The listing builds one solid part. Answer for the finished solid, in the listing's coordinates (mm). A direction names the side the tool comes from. Round coordinates to 2 decimals unless told otherwise and drop trailing zeros. Write each loop counter-clockwise with the first axis right and the second up, starting at its lowest first coordinate (ties: lowest second). Pieces come first, ordered by that corner, then holes. Notation, with made-up numbers: M -26,89 L -9,89 A24 ccw -9,114 Z; hole C 71,-21 d11. An arc over 180 degrees is marked long. One line per item, written item: value. Start each with the question number.
(1) Section A-A (y = -18.5) is taken. Determine the outline of the cut face in (x, z), plus the area to 3 significant figures.
(2) Given P1, Ø7, axis at x = -23.5, y = 2.5, coming from the +Z side; P2, Ø13, axis at y = -3.5, z = 44, coming from the -X side; P3, Ø3, axis at x = -89, z = 44.5, coming from the +Y side; P4, Ø2, axis at x = -117, y = 0, coming from the -Z side, each flat-ended and moving along its own axis, determine where each tip first touches the part or whether it passes through.
(3) Section C-C (x = -32.5) is taken. Determine the outline of the cut face in (y, z).
(4) For faces 4 (the flat face through (-37, -5, 8)), 5 (the flat face through (-89, -13, 36)), 6 (the flat face through (-40.414, -18.944, 40.326)), 7 (the flat face through (-213.75, 4, 4)), 8 (the flat face through (-109, -8, 8)), determine the directions among +Z, -Z, +X, -X, +Y, -Y from which every point of the face is accessible in a straight line to the end or side of a thin tool.
(5) For a pull along Z with two mould halves and no side action, classify faces 1 (the flat face through (-52, -15, 17)), 2 (the cylindrical face through (-146.203, -19.056, 19.141)), 3 (the flat face through (-133, -6, 43)) as released by +Z, released by -Z, zero draft, split by the parting line, or undercut.
(6) Consider probe 1 along X at (y, z) = (-5, 20); probe 2 along X at (y, z) = (-17.5, 37.5); probe 3 along Y at (x, z) = (-143, 15). Determine where each line is inside the solid, lowest interval first.
(7) Section B-B (z = 40) is taken. Determine the outline of the cut face in (x, y).
(8) Section D-D (x = -218) is taken. Determine the outline of the cut face in (y, z).
```python
from build123d import *

# Parameters (mm, degrees)
BOSS_EXTRUDE1_DEPTH = 8
BOSS_EXTRUDE2_DEPTH = 8
BOSS_EXTRUDE3_DEPTH = 8
BOSS_EXTRUDE4_DEPTH = 8
SKETCH6_W           = 40
SKETCH6_H           = 52
CUT_EXTRUDE1_DEPTH  = 9
CUT_EXTRUDE2_DEPTH  = 9
FILLET1_R           = 4
FILLET2_R           = 2
FILLET3_R           = 4
FILLET4_R           = 3
FILLET5_R           = 2


with BuildPart() as part:
    # Sketch1 → Boss-Extrude1 (new body)
    with BuildSketch(Plane.XY):
        with BuildLine():
            Line((4.25, 9), (4.25, 0))
            ThreePointArc((4.25, 0), (0, -4.25), (-4.25, 0))
            Line((-4.25, 0), (-4.25, 9))
            Line((-4.25, 9), (-12.5, 9))
            Line((-12.5, 9), (-18.5, 3))
            Line((-18.5, 3), (-89, 3))
            Line((-89, 3), (-92, 0))
            Line((-92, 0), (-126, 0))
            Line((-126, 0), (-129, 3))
            Line((-129, 3), (-199.5, 3))
            Line((-199.5, 3), (-205.5, 9))
            Line((-205.5, 9), (-213.75, 9))
            Line((-213.75, 9), (-213.75, 0))
            ThreePointArc((-213.75, 0), (-218, -4.25), (-222.25, 0))
            Line((-222.25, 0), (-222.25, 9))
            Line((-222.25, 9), (-227, 9))
            Line((-227, 9), (-227, -23))
            Line((-227, -23), (9, -23))
            Line((9, -23), (9, 9))
            Line((9, 9), (4.25, 9))
        make_face()
    extrude(amount=BOSS_EXTRUDE1_DEPTH)

    # Sketch2 → Boss-Extrude2 (add)
    with BuildSketch(Plane.XZ.offset(23)):
        Polygon((-227, 8), (-227, 16), (-137, 78), (-81, 78), (9, 16), (9, 8), align=None)
    extrude(amount=-BOSS_EXTRUDE2_DEPTH)

    # Sketch4 → Boss-Extrude3 (add)
    with BuildSketch(Plane(origin=(-81, 0, 0), x_dir=(0, 0, -1), z_dir=(1, 0, 0))):
        Polygon((-78, -15), (-8, 3), (-8, 0), (-8, -15), align=None)
    extrude(amount=-BOSS_EXTRUDE3_DEPTH)

    # Sketch5 → Boss-Extrude4 (add)
    with BuildSketch(Plane(origin=(-137, 0, 0), x_dir=(0, 0, -1), z_dir=(1, 0, 0))):
        Polygon((-8, 3), (-78, -15), (-8, -15), (-8, 0), align=None)
    extrude(amount=BOSS_EXTRUDE4_DEPTH)

    # Sketch6 → Cut-Extrude1 (cut, through all)
    with BuildSketch(Plane(origin=(0, -15, 0), x_dir=(1, 0, 0), z_dir=(0, 1, 0))):
        with Locations((-109, -44)):
            Rectangle(SKETCH6_W, SKETCH6_H)
    extrude(amount=-CUT_EXTRUDE1_DEPTH, mode=Mode.SUBTRACT)

    # Sketch7 → Cut-Extrude2 (cut, through all)
    with BuildSketch(Plane(origin=(0, -15, 0), x_dir=(1, 0, 0), z_dir=(0, 1, 0))):
        Polygon((-73, -18), (-8.004981773, -18), (-73, -62.77434589), align=None)
        Polygon((-145, -18), (-209.995018227, -18), (-145, -62.77434589), align=None)
    extrude(amount=-CUT_EXTRUDE2_DEPTH, mode=Mode.SUBTRACT)

    # Fillet1
    fillet1_edges = [part.edges().sort_by_distance(p)[0] for p in [
        (-129, -19, 18),
        (-89, -19, 18),
        (-73, -19, 18),
        (-145, -19, 18),
    ]]
    fillet(fillet1_edges, radius=FILLET1_R)

    # Fillet2
    fillet2_edges = [part.edges().sort_by_distance(p)[0] for p in [
        (-8.004981773, -19, 18),
        (-209.995018227, -19, 18),
    ]]
    fillet(fillet2_edges, radius=FILLET2_R)

    # Fillet3
    fillet3_edges = [part.edges().sort_by_distance(p)[0] for p in [
        (-129, -19, 70),
        (-89, -19, 70),
    ]]
    fillet(fillet3_edges, radius=FILLET3_R)

    # Fillet4
    fillet4_edges = [part.edges().sort_by_distance(p)[0] for p in [
        (-73, -19, 62.77434589),
        (-145, -19, 62.77434589),
    ]]
    fillet(fillet4_edges, radius=FILLET4_R)

    # Fillet5
    fillet5_edges = [part.edges().sort_by_distance(p)[0] for p in [
        (9, 9, 4),
        (4.25, 9, 4),
        (-4.25, 9, 4),
        (-213.75, 9, 4),
        (-222.25, 9, 4),
        (-227, 9, 4),
    ]]
    fillet(fillet5_edges, radius=FILLET5_R)


solid = part.part
```
Recorded:
1. outline: M -227,0 L 9,0 L 9,16 L -81,78 L -137,78 L -227,16 Z; hole M -204.7,21.65 A2 ccw -203.57,18 L -149,18 A4 ccw -145,22 L -145,57.06 A3 ccw -149.7,59.54 Z; hole M -129,22 A4 ccw -125,18 L -93,18 A4 ccw -89,22 L -89,66 A4 ccw -93,70 L -125,70 A4 ccw -129,66 Z; hole M -73,22 A4 ccw -69,18 L -14.43,18 A2 ccw -13.3,21.65 L -68.3,59.54 A3 ccw -73,57.06 Z
1. area: 7,890 mm2
2. P1: stops at z = 8
2. P2: stops at x = -137
2. P3: stops at y = -6
2. P4: stops at z = 0
3. outline: M -23,0 L 3,0 L 3,8 L -15,8 L -15,18 L -23,18 Z; M -23,34.87 L -15,34.87 L -15,44.59 L -23,44.59 Z
4. face 4: +Z, +X, +Y
4. face 5: +Y
4. face 6: +Y, -Y
4. face 7: +Z, -Z, +Y
4. face 8: +Z, +Y
5. face 1: zero draft
5. face 2: undercut
5. face 3: released by +Z
6. probe 1: x = -137 to -129, -89 to -81
6. probe 2: x = -195.79 to -181.69, -145 to -129, -89 to -73, -36.31 to -22.21
6. probe 3: y = -23 to -15
7. outline: M -192.16,-23 L -178.06,-23 L -178.06,-15 L -192.16,-15 Z; M -145,-23 L -129,-23 L -129,-5.23 L -137,-5.23 L -137,-15 L -145,-15 Z; M -89,-23 L -73,-23 L -73,-15 L -81,-15 L -81,-5.23 L -89,-5.23 Z; M -39.94,-23 L -25.84,-23 L -25.84,-15 L -39.94,-15 Z
8. outline: M -23,0 L -4.25,0 L -4.25,8 L -15,8 L -15,22.2 L -23,22.2 Z
